```python
from build123d import *

# Parameters (mm, degrees)
EXTRUDE_DEPTH    = 2
EXTRUDE001_DEPTH = 2
EXTRUDE002_DEPTH = 2
BOX009_W         = 226
BOX009_H         = 17
BOX009_DEPTH     = 2
BOX015_W         = 10
BOX015_H         = 3
BOX015_DEPTH     = 10
BOX010_W         = 3
BOX010_H         = 13.5
BOX010_DEPTH     = 15
BOX022_W         = 30
BOX022_H         = 2
BOX022_DEPTH     = 6
BOX023_W         = 6
BOX023_H         = 2
BOX023_DEPTH     = 20
BOX001_W         = 180
BOX001_H         = 34
BOX001_DEPTH     = 98
BOX_W            = 226
BOX_H            = 2
BOX_DEPTH        = 118


with BuildPart() as top_thin_beam:
    # Sketch (on Sketch) → Extrude (new body)
    with BuildSketch(Plane.XY):
        Polygon((0, 0), (0, 6.3), (26, 4.5), (204, 4.5), (230, 6.3), (230, 0), align=None)
    extrude(amount=EXTRUDE_DEPTH)


with BuildPart() as top_thin_beam_1:
    # Extrude placement: moved
    add(top_thin_beam.part.moved(Location((0, 0, 116))))


with BuildPart() as rightverticalcontour:
    # Sketch001 → Extrude001 (new body)
    with BuildSketch(Plane.YZ):
        Polygon((0, 0), (15, 0), (15, 56), (11, 56), (15, 90), (15, 104), (11, 113), (6.3, 118), (0, 118), align=None)
    extrude(amount=EXTRUDE001_DEPTH)


with BuildPart() as rightverticalcontour_1:
    # Extrude001 placement: moved
    add(rightverticalcontour.part.moved(Location((228, 0, 0))))


with BuildPart() as obj1:
    # Sketch002 → Extrude002 (new body)
    with BuildSketch(Plane.YZ):
        Polygon((0, 0), (15, 0), (15, 56), (11, 56), (15, 90), (15, 104), (11, 113), (6.3, 118), (0, 118), align=None)
    extrude(amount=EXTRUDE002_DEPTH)


with BuildPart() as bottom:
    # Box009 → Box009 (new body)
    with BuildSketch(Plane(origin=(2, 0, 0), x_dir=(1, 0, 0), z_dir=(0, 0, 1))):
        with Locations((113, 8.5)):
            Rectangle(BOX009_W, BOX009_H)
    extrude(amount=BOX009_DEPTH)


with BuildPart() as slot:
    # Box015 → Box015 (new body)
    with BuildSketch(Plane(origin=(-3.5, 7.5, 7.5), x_dir=(1, 0, 0), z_dir=(0, 0, 1))):
        with Locations((5, 1.5)):
            Rectangle(BOX015_W, BOX015_H)
    extrude(amount=BOX015_DEPTH)


with BuildPart() as base:
    # Box010 → Box010 (new body)
    with BuildSketch(Plane.XY):
        with Locations((1.5, 6.75)):
            Rectangle(BOX010_W, BOX010_H)
    extrude(amount=BOX010_DEPTH)


with BuildPart() as topleftbacksupport:
    # Cut001 base: copy of base
    add(base.part)

    # Cut001: cut slot
    add(slot.part, mode=Mode.SUBTRACT)


with BuildPart() as topleftbacksupport_1:
    # Cut001 placement: moved
    add(topleftbacksupport.part.moved(Location((9, 2, 79.25))))


with BuildPart() as bottomleftbacksupport:
    # Cut002 base: copy of base
    add(base.part)

    # Cut002: cut slot
    add(slot.part, mode=Mode.SUBTRACT)


with BuildPart() as bottomleftbacksupport_1:
    # Cut002 placement: moved
    add(bottomleftbacksupport.part.moved(Location((9, 2, 22.75))))


with BuildPart() as bottomrightbacksupport:
    # Cut003 base: copy of base
    add(base.part)

    # Cut003: cut slot
    add(slot.part, mode=Mode.SUBTRACT)


with BuildPart() as bottomrightbacksupport_1:
    # Cut003 placement: moved
    add(bottomrightbacksupport.part.moved(Location((212, 2, 22.75))))


with BuildPart() as toprightbacksupport:
    # Cut004 base: copy of base
    add(base.part)

    # Cut004: cut slot
    add(slot.part, mode=Mode.SUBTRACT)


with BuildPart() as toprightbacksupport_1:
    # Cut004 placement: moved
    add(toprightbacksupport.part.moved(Location((212, 2, 79.25))))


with BuildPart() as bottomcableguard:
    # Box022 → Box022 (new body)
    with BuildSketch(Plane(origin=(187, 15, 2), x_dir=(1, 0, 0), z_dir=(0, 0, 1))):
        with Locations((15, 1)):
            Rectangle(BOX022_W, BOX022_H)
    extrude(amount=BOX022_DEPTH)


with BuildPart() as sidecableguard:
    # Box023 → Box023 (new body)
    with BuildSketch(Plane(origin=(222, 13, 12), x_dir=(1, 0, 0), z_dir=(0, 0, 1))):
        with Locations((3, 1)):
            Rectangle(BOX023_W, BOX023_H)
    extrude(amount=BOX023_DEPTH)


with BuildPart() as cube001:
    # Box001 → Box001 (new body)
    with BuildSketch(Plane(origin=(25, -17, 10), x_dir=(1, 0, 0), z_dir=(0, 0, 1))):
        with Locations((90, 17)):
            Rectangle(BOX001_W, BOX001_H)
    extrude(amount=BOX001_DEPTH)


with BuildPart() as fusion:
    # Box → Box (new body)
    with BuildSketch(Plane(origin=(2, 0, 0), x_dir=(1, 0, 0), z_dir=(0, 0, 1))):
        with Locations((113, 1)):
            Rectangle(BOX_W, BOX_H)
    extrude(amount=BOX_DEPTH)

    # Cut: cut Cube001
    add(cube001.part, mode=Mode.SUBTRACT)

    # Fusion: union Top Thin Beam, RightVerticalContour, obj1, Bottom, TopLeftBackSupport, BottomLeftBackSupport, BottomRightBackSupport, TopRightBackSupport, BottomCableGuard, SideCableGuard
    add(top_thin_beam_1.part)
    add(rightverticalcontour_1.part)
    add(obj1.part)
    add(bottom.part)
    add(topleftbacksupport_1.part)
    add(bottomleftbacksupport_1.part)
    add(bottomrightbacksupport_1.part)
    add(toprightbacksupport_1.part)
    add(bottomcableguard.part)
    add(sidecableguard.part)


solid = fusion.part
```
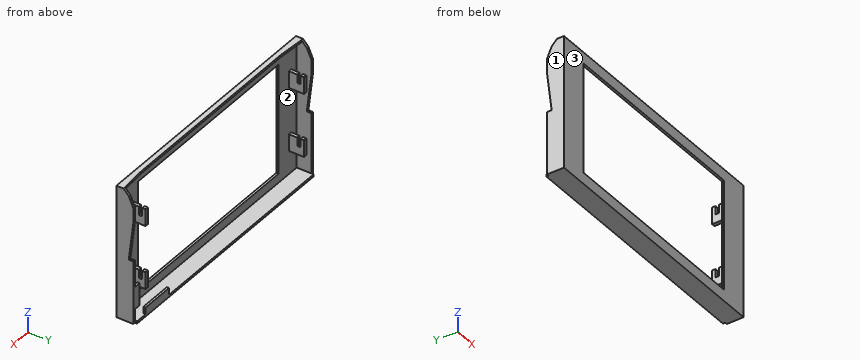
Work out the finished part from the listing and answer in its coordinate system (mm). Face numbers are marked on the shaded views. Round coordinates to 2 decimals unless told otherwise and drop trailing zeros. Write each loop counter-clockwise with the first axis right and the second up, starting at its lowest first coordinate (ties: lowest second). Pieces come first, ordered by that corner, then holes.
1) A cutting plane is placed at C-C on x = 18. Determine the outline of the cut face in (y, z), and give its area (3 significant figures).
2) Flat-ended cylindrical pins translate along their axes: P1, Ø5, axis at x = 43.5, y = 7.5, coming from the +Z side; P2, Ø1.5, axis at x = 11, y = 11.5, coming from the +Z side; P3, Ø1.6, axis at x = 228.5, z = 94, coming from the +Y side; P4, Ø2, axis at y = 10.5, z = 57.5, coming from the -X side. Find the tip coordinate at first contact, or state that the pin passes through.
3) A cutting plane is placed at A-A on z = 51.5. Determine the outline of the cut face in (x, y), and give its area (3 significant figures).
4) Determine the mould class of the marked faces 1, 2 and 3 for opening direction X: pulls with the +X half, pulls with the -X half, needs draft (parallel to the pull), parting line crosses it, or undercut.
5) Consider probe 1 along X at (y, z) = (5, 92); probe 2 along X at (y, z) = (8.5, 13.5); probe 3 along X at (y, z) = (14.25, 29.5). Determine where each line is inside the solid, lowest interval first.
6) A cutting plane is placed at B-B on x = 146. Determine the outline of the cut face in (y, z).
Entries:
1. outline: (0, 0) - (17, 0) - (17, 2) - (2, 2) - (2, 116) - (5.05, 116) - (5.05, 118) - (0, 118) - close
1. area: 272 mm2
2. P1: stops at z = 2
2. P2: stops at z = 86.75
2. P3: stops at y = 15
2. P4: stops at x = 0
3. outline: (0, 0) - (25, 0) - (25, 2) - (2, 2) - (2, 15) - (0, 15) - close; (205, 0) - (230, 0) - (230, 15) - (228, 15) - (228, 2) - (205, 2) - close
3. area: 152 mm2
4. face 1: pulls with the -X half
4. face 2: undercut
4. face 3: needs draft
5. probe 1: x = 0 to 2, 9 to 12, 212 to 215, 228 to 230
5. probe 2: x = 0 to 2, 228 to 230
5. probe 3: x = 0 to 2, 9 to 12, 212 to 215, 222 to 230
6. outline: (0, 0) - (17, 0) - (17, 2) - (2, 2) - (2, 10) - (0, 10) - close; (0, 108) - (2, 108) - (2, 116) - (4.5, 116) - (4.5, 118) - (0, 118) - close
